from build123d import *

# Parameters (mm, degrees)
SKETCH2_W           = 60
SKETCH2_H           = 60
SKETCH2_R           = 2.5
SKETCH2_R_2         = 21.05
BOSS_EXTRUDE1_DEPTH = 3
FILLET1_R           = 3


with BuildPart() as part:
    # Sketch2 → Boss-Extrude1 (new body)
    with BuildSketch(Plane.XY):
        with Locations((10.311464729, 39.343711654)):
            Rectangle(SKETCH2_W, SKETCH2_H)
        with Locations((33.881464729, 15.773711654)):
            Circle(SKETCH2_R, mode=Mode.SUBTRACT)
        with Locations((-13.258535271, 15.773711654)):
            Circle(SKETCH2_R, mode=Mode.SUBTRACT)
        with Locations((-13.258535271, 62.913711654)):
            Circle(SKETCH2_R, mode=Mode.SUBTRACT)
        with Locations((10.311464729, 39.343711654)):
            Circle(SKETCH2_R_2, mode=Mode.SUBTRACT)
        with Locations((33.881464729, 62.913711654)):
            Circle(SKETCH2_R, mode=Mode.SUBTRACT)
    extrude(amount=BOSS_EXTRUDE1_DEPTH)

    # Fillet1
    fillet1_edges = [part.edges().sort_by_distance(p)[0] for p in [
        (-19.688535271, 9.343711654, 1.5),
        (-19.688535271, 69.343711654, 1.5),
        (40.311464729, 69.343711654, 1.5),
        (40.311464729, 9.343711654, 1.5),
    ]]
    fillet(fillet1_edges, radius=FILLET1_R)


solid = part.part
Here's how the part is built. I have some questions about the finished solid (model axes, mm). Coordinates: 2 decimals unless noted, no trailing zeros. Order: outer loops, then holes, each group sorted by start corner. A loop starts at its lowest first (then second) coordinate and runs counter-clockwise, first axis right, second up. Notation, with made-up numbers: M 53,16 L 79,16 A31 cw 79,55 Z; hole C -28,81.5 d10. An arc over 180 degrees is marked long. Answer as CSV lines item,"result". Start each with the question number.
1. I need wall thicknesses on line 1 (Y direction, x = -13.5, z = 2.7); line 2 (X direction, y = 13.5, z = 2); line 3 (Y direction, x = -11, z = 1.3). Which ranges of each line are inside material? Lowest first, please. Write a range as [from, to].
2. I want a section at C-C, the plane x = 34. Write out the boundary of the cut face in (y, z).
3. I want a section at D-D, the plane z = 0.8. Write out the boundary of the cut face in (x, y).
4. I want a section at B-B, the plane y = 30.5. Write out the boundary of the cut face in (x, z), and give its area (3 significant figures).
5. I want a section at A-A, the plane x = 11. Write out the boundary of the cut face in (y, z).
6. We'd pull the mould along Y, two halves only. Please class faces 1 (the cylindrical face through (36.191, 14.816, 1.479)), 2 (the cylindrical face through (-18.833, 10.246, 1.521)), 3 (the flat face through (-19.689, 39, 1)): released by +Y, released by -Y, zero draft, split by the parting line, or undercut.
Recorded:
1,line 1,"y = [9.34, 13.29], [18.26, 60.43], [65.4, 69.34]"
1,line 2,"x = [-19.69, -14.3], [-12.22, 32.84], [34.92, 40.31]"
1,line 3,"y = [9.34, 14.7], [16.85, 61.84], [63.99, 69.34]"
2,outline,"M 9.34,0 L 13.28,0 L 13.28,3 L 9.34,3 Z; M 18.27,0 L 60.42,0 L 60.42,3 L 18.27,3 Z; M 65.41,0 L 69.34,0 L 69.34,3 L 65.41,3 Z"
3,outline,"M -19.69,12.34 A3 ccw -16.69,9.34 L 37.31,9.34 A3 ccw 40.31,12.34 L 40.31,66.34 A3 ccw 37.31,69.34 L -16.69,69.34 A3 ccw -19.69,66.34 Z; hole C -13.26,15.77 d5; hole C -13.26,62.91 d5; hole C 10.31,39.34 d42.1; hole C 33.88,15.77 d5; hole C 33.88,62.91 d5"
4,outline,"M -19.69,0 L -8.79,0 L -8.79,3 L -19.69,3 Z; M 29.41,0 L 40.31,0 L 40.31,3 L 29.41,3 Z"
4,area,"65.4 mm2"
5,outline,"M 9.34,0 L 18.3,0 L 18.3,3 L 9.34,3 Z; M 60.38,0 L 69.34,0 L 69.34,3 L 60.38,3 Z"
6,face 1,"undercut"
6,face 2,"released by -Y"
6,face 3,"zero draft"
